Verification items for the finished model (mm, model axes). A direction names the side the tool comes from. Coordinates: 2 decimals unless noted, no trailing zeros. Write each loop counter-clockwise with the first axis right and the second up, starting at its lowest first coordinate (ties: lowest second). Pieces come first, ordered by that corner, then holes. Notation, with made-up numbers: M -13.5,-29.5 L 15.5,-29.5 A13 ccw 15.5,-21.5 Z; hole C 69.5,-26.5 d6. An arc over 180 degrees is marked long. One line per item, written item: value.
```python
from build123d import *

# Parameters (mm, degrees)
SKETCH001_R   = 1.5
SKETCH001_R_2 = 1.375
PAD001_DEPTH  = 1.5
FILLET001_R   = 0.2
FILLET002_R   = 0.2
FILLET003_R   = 0.2


with BuildPart() as part:
    # Sketch001 → Pad001 (new body)
    with BuildSketch(Plane.XY):
        with BuildLine():
            Line((-35.07682, -14.822674), (35.499554, -14.822674))
            ThreePointArc((35.499554, -14.822674), (36.206661, -14.529781), (36.499554, -13.822674))
            Line((36.499554, -13.822674), (36.499554, 14.149868))
            ThreePointArc((36.499554, 14.149868), (36.206661, 14.856975), (35.499554, 15.149868))
            Line((35.499554, 15.149868), (-35.07682, 15.149868))
            ThreePointArc((-35.07682, 15.149868), (-35.783927, 14.856975), (-36.07682, 14.149868))
            Line((-36.07682, 14.149868), (-36.07682, -13.822674))
            ThreePointArc((-36.07682, -13.822674), (-35.783927, -14.529781), (-35.07682, -14.822674))
        make_face()
        with Locations((-31.664087, -11.774244)):
            Circle(SKETCH001_R, mode=Mode.SUBTRACT)
        with Locations((-31.670164, 11.730007)):
            Circle(SKETCH001_R, mode=Mode.SUBTRACT)
        with Locations((-7.183492, -11.791598)):
            Circle(SKETCH001_R, mode=Mode.SUBTRACT)
        with Locations((-7.228608, 11.705488)):
            Circle(SKETCH001_R, mode=Mode.SUBTRACT)
        with Locations((32.976643, 10.303188)):
            Circle(SKETCH001_R_2, mode=Mode.SUBTRACT)
        with Locations((33.041733, -10.508623)):
            Circle(SKETCH001_R_2, mode=Mode.SUBTRACT)
        with BuildLine():
            Line((34.398702, 8.193074), (23.707742, 8.193074))
            ThreePointArc((23.707742, 8.193074), (22.498043, 7.692), (21.996969, 6.482301))
            Line((21.996969, 6.482301), (21.996969, -6.241538))
            ThreePointArc((21.996969, -6.241538), (22.498043, -7.451237), (23.707742, -7.95231))
            Line((23.707742, -7.95231), (34.398702, -7.95231))
            ThreePointArc((34.398702, -7.95231), (35.608401, -7.451237), (36.109474, -6.241538))
            Line((36.109474, -6.241538), (36.109474, 6.482301))
            ThreePointArc((36.109474, 6.482301), (35.608401, 7.692), (34.398702, 8.193074))
        make_face(mode=Mode.SUBTRACT)
        with BuildLine():
            Line((-30.005591, 12.366703), (-30.005591, -12.32248))
            ThreePointArc((-30.005591, -12.32248), (-29.687046, -13.091518), (-28.918008, -13.410063))
            Line((-28.918008, -13.410063), (-10.086485, -13.410063))
            ThreePointArc((-10.086485, -13.410063), (-9.317448, -13.091518), (-8.998902, -12.32248))
            Line((-8.998902, -12.32248), (-8.998902, 12.366703))
            ThreePointArc((-8.998902, 12.366703), (-9.317448, 13.13574), (-10.086485, 13.454286))
            Line((-10.086485, 13.454286), (-28.918008, 13.454286))
            ThreePointArc((-28.918008, 13.454286), (-29.687046, 13.13574), (-30.005591, 12.366703))
        make_face(mode=Mode.SUBTRACT)
    extrude(amount=PAD001_DEPTH)

    # Fillet001
    fillet001_edges = [part.edges().sort_by_distance(p)[0] for p in [
        (0.211367, -14.822674, 1.5),
    ]]
    fillet(fillet001_edges, radius=FILLET001_R)

    # Fillet002
    fillet002_edges = [part.edges().sort_by_distance(p)[0] for p in [
        (0.211367, -14.822674, 0),
    ]]
    fillet(fillet002_edges, radius=FILLET002_R)

    # Fillet003
    fillet003_edges = [part.edges().sort_by_distance(p)[0] for p in [
        (-30.005591, 0.022111, 1.5),
    ]]
    fillet(fillet003_edges, radius=FILLET003_R)


solid = part.part
```
Item 1: Cross-section at D-D, the plane x = 25.5. Enter the section's corners in (y, z), and give its area (3 significant figures).
The answers:
outline: M -14.82,0.2 A0.2 ccw -14.62,0 L -7.95,0 L -7.95,1.5 L -14.62,1.5 A0.2 ccw -14.82,1.3 Z; M 8.19,0 L 14.95,0 A0.2 ccw 15.15,0.2 L 15.15,1.3 A0.2 ccw 14.95,1.5 L 8.19,1.5 Z
area: 20.7 mm²
Item 2: Cross-section at C-C, the plane z = 0.9. Give the number of separate pieces and of enclosed holes in the cut face, and give its area (3 significant figures).
The answers:
separate pieces: 1
enclosed holes: 8
area: 1,350 mm²
Item 3: Go/stop test with a flat-tipped pin: P1, Ø1.8, axis at x = -31.66, y = -11.77, coming from the +Z side. Record where the tip stops, or that it passes through.
The answers:
P1: passes through
Item 4: Scan lines: line 1 (X direction, y = 4.5, z = 0.3); line 2 (Y direction, x = 33, z = 0.2); line 3 (Y direction, x = 31, z = 0.7). Record each from-to range of solid material in increasing order.
The answers:
line 1: x = -36.08 to -30.01, -9 to 22, 36.11 to 36.5
line 2: y = -14.82 to -11.88, -9.13 to -7.95, 8.19 to 8.93, 11.68 to 15.15
line 3: y = -14.82 to -7.95, 8.19 to 15.15
Item 5: Access from +Z, -Z, +X, -X, +Y, -Y to the whole of each face (thin tool, end or side, straight path). Record for faces 1 (the face through (36.109, 0, 1)), 2 (the face through (0, 0, 0)).
The answers:
face 1: +Z, -Z
face 2: -Z, +X, -X, +Y, -Y
Item 6: Cross-section at A-A, the plane y = -3. Enter the section's corners in (x, z).
The answers:
outline: M -36.08,0.2 A0.2 ccw -35.88,0 L -30.01,0 L -30.01,1.3 A0.2 ccw -30.21,1.5 L -35.88,1.5 A0.2 ccw -36.08,1.3 Z; M -9,0 L 22,0 L 22,1.5 L -8.8,1.5 A0.2 ccw -9,1.3 Z; M 36.11,0 L 36.3,0 A0.2 ccw 36.5,0.2 L 36.5,1.3 A0.2 ccw 36.3,1.5 L 36.11,1.5 Z
Item 7: Draft check along Y on faces 3 (the face through (0, 0, 1.5)), 4 (the face through (35.6, 7.7, 0.7)). Enter one of: released by +Y, released by -Y, zero draft, split by the parting line, or undercut.
The answers:
face 3: zero draft
face 4: undercut
Item 8: Cross-section at B-B, the plane x = -23. Enter the section's corners in (y, z), and give its area (3 significant figures).
The answers:
outline: M -14.82,0.2 A0.2 ccw -14.62,0 L -13.41,0 L -13.41,1.3 A0.2 ccw -13.61,1.5 L -14.62,1.5 A0.2 ccw -14.82,1.3 Z; M 13.45,0 L 14.95,0 A0.2 ccw 15.15,0.2 L 15.15,1.3 A0.2 ccw 14.95,1.5 L 13.65,1.5 A0.2 ccw 13.45,1.3 Z
area: 4.61 mm²
